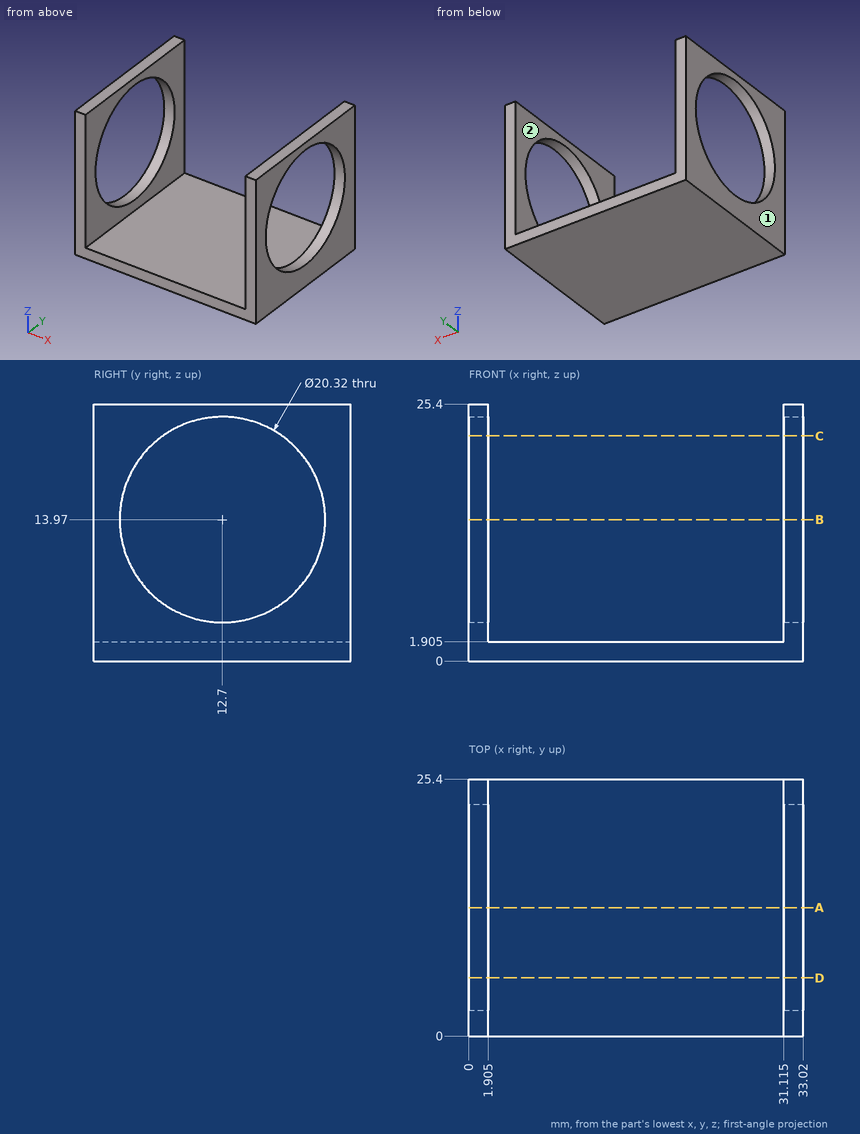
Design review of the part shown in the three views and the two pictorial views. Dimensions are in mm from the part's minimum x, y and z. A direction names the side the tool comes from. Coordinates: 2 decimals unless noted, no trailing zeros. Write each loop counter-clockwise with the first axis right and the second up, starting at its lowest first coordinate (ties: lowest second). Pieces come first, ordered by that corner, then holes.
(1) Add section D-D on y = 5.75. Give the boundary of the cut face in (x, z) (3 decimals).
(2) Add section B-B on z = 13.97. Give the boundary of the cut face in (x, y) (3 decimals), then the cut area to 3 significant figures.
(3) Wall thickness on probe 1 along Z at (x, y) = (1.5, 12.7); probe 2 along X at (y, z) = (16.5, 2.75) (3 decimals); probe 3 along Z at (x, y) = (20, 18) (3 decimals): over which ranges is each line inside the solid? List them lowest first.
(4) Tool access review of the marked faces 1 and 2: name each direction out of +Z, -Z, +X, -X, +Y, -Y from which nothing blocks a thin tool from reaching the whole face with its end or side.
(5) Add section A-A on y = 12.7. Give the boundary of the cut face in (x, z) (3 decimals), then the cut area to 3 significant figures.
(6) For pin 1 Ø12.5 at (x, y) = (13.5, 17) entering from +Z (3 decimals), flat-tipped, find the tip position at first contact; note if it passes through.
(7) Add section C-C on z = 22.25. Give the boundary of the cut face in (x, y) (3 decimals), then the cut area to 3 significant figures.
Answer sheet:
1. outline: (0, 0) - (33.02, 0) - (33.02, 6.559) - (31.115, 6.559) - (31.115, 1.905) - (1.905, 1.905) - (1.905, 6.559) - (0, 6.559) - close; (0, 21.381) - (1.905, 21.381) - (1.905, 25.4) - (0, 25.4) - close; (31.115, 21.381) - (33.02, 21.381) - (33.02, 25.4) - (31.115, 25.4) - close
2. outline: (0, 0) - (1.905, 0) - (1.905, 2.54) - (0, 2.54) - close; (0, 22.86) - (1.905, 22.86) - (1.905, 25.4) - (0, 25.4) - close; (31.115, 0) - (33.02, 0) - (33.02, 2.54) - (31.115, 2.54) - close; (31.115, 22.86) - (33.02, 22.86) - (33.02, 25.4) - (31.115, 25.4) - close
2. area: 19.4 mm2
3. probe 1: z = 0 to 3.81, 24.13 to 25.4
3. probe 2: x = 0 to 1.905, 31.115 to 33.02
3. probe 3: z = 0 to 1.905
4. face 1: +Z, -Z, -X, +Y, -Y
4. face 2: +Z, +Y, -Y
5. outline: (0, 0) - (33.02, 0) - (33.02, 3.81) - (31.115, 3.81) - (31.115, 1.905) - (1.905, 1.905) - (1.905, 3.81) - (0, 3.81) - close; (0, 24.13) - (1.905, 24.13) - (1.905, 25.4) - (0, 25.4) - close; (31.115, 24.13) - (33.02, 24.13) - (33.02, 25.4) - (31.115, 25.4) - close
5. area: 75.0 mm2
6. pin 1: stops at z = 1.905
7. outline: (0, 0) - (1.905, 0) - (1.905, 6.812) - (0, 6.812) - close; (0, 18.588) - (1.905, 18.588) - (1.905, 25.4) - (0, 25.4) - close; (31.115, 0) - (33.02, 0) - (33.02, 6.812) - (31.115, 6.812) - close; (31.115, 18.588) - (33.02, 18.588) - (33.02, 25.4) - (31.115, 25.4) - close
7. area: 51.9 mm2
